Here's how the part is built. I have some questions about the finished solid (model axes, mm). Face numbers are marked on the shaded views. A direction names the side the tool comes from. Round coordinates to 2 decimals unless told otherwise and drop trailing zeros. Order: outer loops, then holes, each group sorted by start corner. A loop starts at its lowest first (then second) coordinate and runs counter-clockwise, first axis right, second up. Notation, with made-up numbers: (-36, 67) - (4, 67) arc R25 cw to (4, 89) - close; hole circle Ø2 at (-2.75, -24.5). An arc over 180 degrees is marked (long way). One line per item, written item: value.
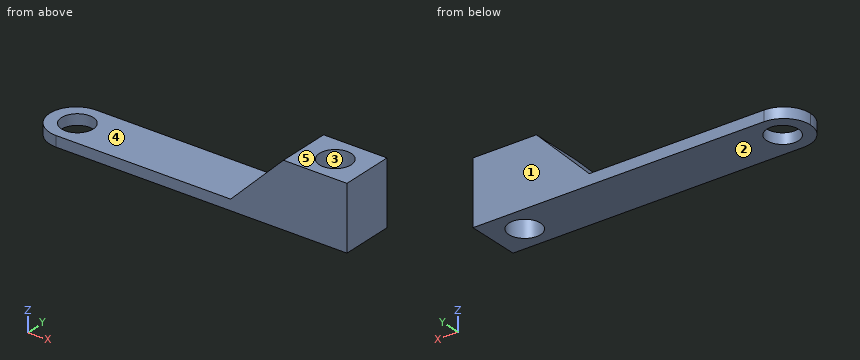
from build123d import *

# Parameters (mm, degrees)
F1_DEPTH = 12.5
F2_R     = 7.5
F3_DEPTH = 30
F5_R     = 12.49999
F4_R     = 7.5
F6_DEPTH = 5


# Not quite as in the source:
# - a fillet or chamfer is up to 0.001 mm smaller than in the source, because OpenCascade refuses the exact size


with BuildPart() as f1:
    # F0 (on Front) → F1 (new body, symmetric)
    with BuildSketch(Plane.XZ):
        Polygon((-150, 0), (0, 0), (0, 30), (-30, 30), (-55, 5), (-150, 5), align=None)
    extrude(amount=F1_DEPTH, both=True)

    # F2 (on face) → F3 (cut, through all)
    with BuildSketch(Plane.XY.offset(30)):
        with Locations((-15, 0)):
            Circle(F2_R)
    extrude(amount=-F3_DEPTH, mode=Mode.SUBTRACT)

    # F5 (radius 12.5 in the source; OpenCascade refuses exactly that, so slightly less here)
    f5_edges = [f1.edges().sort_by_distance(p)[0] for p in [
        (-150, 12.5, 2.5),
        (-150, -12.5, 2.5),
    ]]
    fillet(f5_edges, radius=F5_R)

    # F4 (on face) → F6 (cut, through all)
    with BuildSketch(Plane.XY.offset(5)):
        with Locations((-136.9243115187, 0)):
            Circle(F4_R)
    extrude(amount=-F6_DEPTH, mode=Mode.SUBTRACT)


solid = f1.part
Q1. If we section it at B-B, the plane y = 4: Please give me the cut outline in (x, z).
Results list:
outline: (-149.34, 0) - (-143.27, 0) - (-143.27, 5) - (-149.34, 5) - close; (-130.58, 0) - (-21.34, 0) - (-21.34, 30) - (-30, 30) - (-55, 5) - (-130.58, 5) - close; (-8.66, 0) - (0, 0) - (0, 30) - (-8.66, 30) - close
Q2. We'd pull the mould along Y, two halves only. Please class the marked faces 1, 2 and 3: released by +Y, released by -Y, zero draft, split by the parting line, or undercut.
Results list:
face 1: released by +Y
face 2: zero draft
face 3: undercut
Q3. Which directions (+Z, -Z, +X, -X, +Y, -Y) give clear straight access to the entire face, cutting with the end or side of a thin tool? Please do the marked faces 4 and 5.
Results list:
face 4: +Z, -X, +Y, -Y
face 5: +Z, +X, -X, +Y, -Y
Q4. If we section it at D-D, the plane x = -91: Please give me the cut outline in (y, z), then the cut area to 3 significant figures.
Results list:
outline: (-12.5, 0) - (12.5, 0) - (12.5, 5) - (-12.5, 5) - close
area: 125 mm²
Q5. If we section it at A-A, the plane x = -15: Please give me the cut outline in (y, z).
Results list:
outline: (-12.5, 0) - (-7.5, 0) - (-7.5, 30) - (-12.5, 30) - close; (7.5, 0) - (12.5, 0) - (12.5, 30) - (7.5, 30) - close
Q6. If I drill on line 1 along Y through (x, z) = (-15, 12.25); line 2 along X through (y, z) = (6.5, 3.75); line 3 along Z through (x, y) = (-127.5, 10.5), over which ranges is the centre line in solid material (lowest first)?
Results list:
line 1: -12.5 to -7.5, 7.5 to 12.5
line 2: -148.18 to -140.67, -133.18 to -18.74, -11.26 to 0
line 3: 0 to 5
Q7. Will these pins go through, and if not, where does the flat tip stop? pin 1 (13.5 mm diameter, centred on x = -15, y = 0, fed in from -Z); pin 2 (4 mm diameter, centred on x = -95.5, y = -2.5, fed in from +Z).
Results list:
pin 1: through
pin 2: z = 5
Q8. If we section it at C-C, the plane z = 8.5: Please give me the cut outline in (x, y).
Results list:
outline: (-51.5, -12.5) - (0, -12.5) - (0, 12.5) - (-51.5, 12.5) - close; hole circle Ø15 at (-15, 0)
